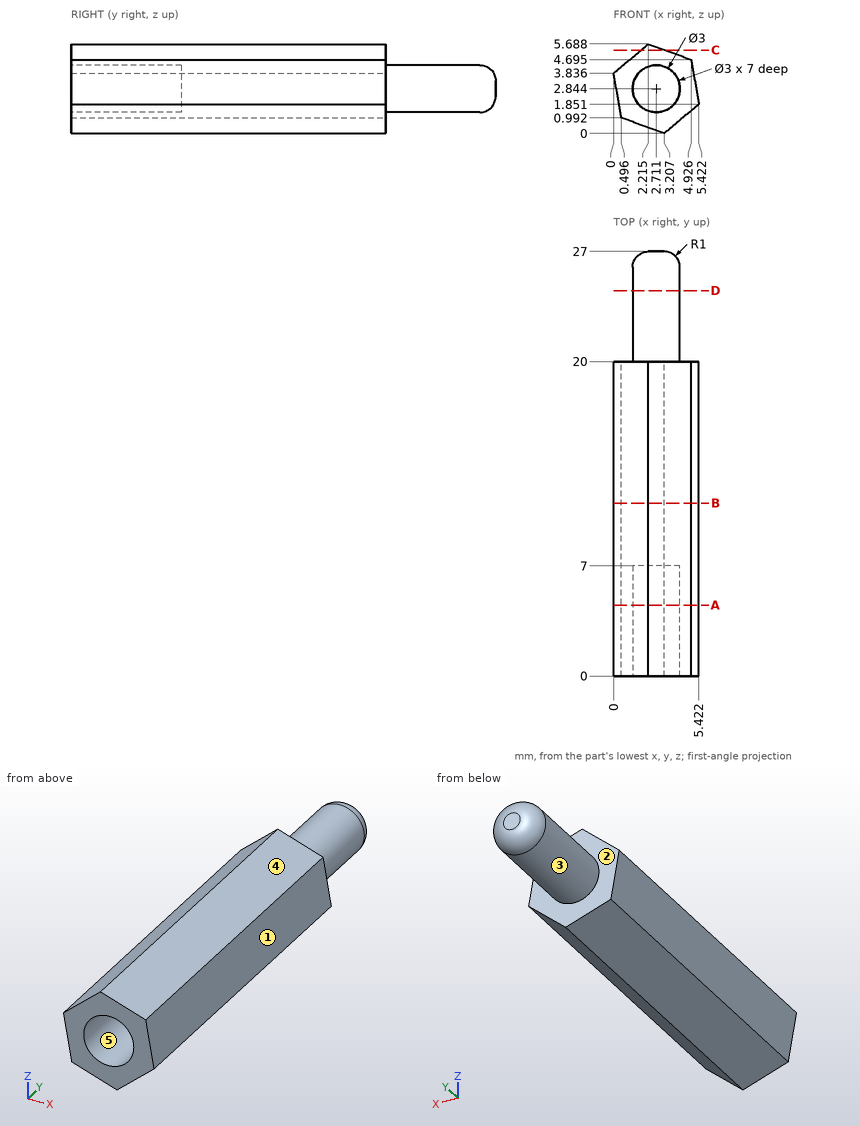
Geometry: see drawing. Coordinates: mm, zero at the bounding-box minimum. A direction names the side the tool comes from. Round coordinates to 2 decimals unless told otherwise and drop trailing zeros. Loops run counter-clockwise (first coordinate to the right, second up) from the corner with the lowest first, then second, coordinate; pieces in that order, holes last. Notation, with made-up numbers: (-33, 81.5) - (-3, 81.5) arc R23 cw to (-3, 96.5) - close; hole circle Ø5 at (-26, 34.5). An arc over 180 degrees is marked (long way). Write item = value, one per line. Start each with the question number.
(1) Section query D-D, the plane y = 24.5. Output: boundary loops of the cut face in (x, z).
(2) Ray query, line 1 along Y through (x, z) = (0.9, 2.1); line 2 along Z through (x, y) = (3.4, 1.5) (1 decimal); line 3 along Z through (x, y) = (2.7, 20.75). Return the intervals inside material, ascending. Write a range as from..to.
(3) Set-up query: the marked faces 1 and 2. Return all of +Z, -Z, +X, -X, +Y, -Y with unobstructed straight access to the full face (end or side cutting, diameter ignored); none if empty.
(4) Pin query (flat end, axial travel): pin 1 (1 mm diameter, centred on y = 6, z = 2.5, fed in from -X); pin 2 (1 mm diameter, centred on x = 1.5, y = 12, fed in from +Z); pin 3 (1 mm diameter, centred on y = 9.5, z = 1.5, fed in from -X). Return the tip coordinate at first contact, or that it passes through.
(5) Section query A-A, the plane y = 4.5. Output: boundary loops of the cut face in (x, z) (1 decimal), plus the area to 3 significant figures.
(6) Pull-direction query (Z, two-part tool) for the marked faces 3, 4 and 5; classes: +Z half, -Z half, draft (parallel to the pull), parting line (faces both ways), or undercut.
(7) Section query C-C, the plane z = 5.3. Output: boundary loops of the cut face in (x, y).
(8) Section query B-B, the plane y = 11. Output: boundary loops of the cut face in (x, z) (1 decimal).
Conclusion:
q1.outline = circle Ø3 at (2.71, 2.84)
q2.line_1 = 0..20
q2.line_2 = 0.2..1.5, 4.2..5.3
q2.line_3 = 1.34..4.34
q3.face_1 = +Z, +X, +Y, -Y
q3.face_2 = +Y
q4.pin_1 = 0.15
q4.pin_2 = 5.51
q4.pin_3 = 0.32
q5.outline = (0, 3.8) - (0.5, 1) - (3.2, 0) - (5.4, 1.9) - (4.9, 4.7) - (2.2, 5.7) - close; hole circle Ø3 at (2.7, 2.8)
q5.area = 14.6 mm2
q6.face_3 = parting line
q6.face_4 = +Z half
q6.face_5 = undercut
q7.outline = (1.75, 0) - (3.27, 0) - (3.27, 20) - (1.75, 20) - close
q8.outline = (0, 3.8) - (0.5, 1) - (3.2, 0) - (5.4, 1.9) - (4.9, 4.7) - (2.2, 5.7) - close
